from build123d import *

# Parameters (mm, degrees)
CROQUIS1_R              = 8.001
SALIENTE_EXTRUIR1_DEPTH = 31.75
SALIENTE_EXTRUIR2_DEPTH = 12.7
CROQUIS3_W              = 47.752
CROQUIS3_H              = 44.704
CORTAR_EXTRUIR4_DEPTH   = 6.35


with BuildPart() as part:
    # Croquis1 → Saliente-Extruir1 (new body)
    with BuildSketch(Plane(origin=(0, 0, 0), x_dir=(1, 0, 0), z_dir=(0, 1, 0))):
        with BuildLine():
            Line((0, -22.352), (25.4, -22.352))
            Line((25.4, -22.352), (25.4, 22.352))
            Line((25.4, 22.352), (0, 22.352))
            ThreePointArc((0, 22.352), (-22.352, 0), (0, -22.352))
        make_face()
        Circle(CROQUIS1_R, mode=Mode.SUBTRACT)
    extrude(amount=SALIENTE_EXTRUIR1_DEPTH)

    # Croquis1<3> → Saliente-Extruir2 (add)
    with BuildSketch(Plane(origin=(0, 0, 0), x_dir=(1, 0, 0), z_dir=(0, 1, 0))):
        with BuildLine():
            Line((69.85, -22.352), (69.85, -6.35))
            Line((69.85, -6.35), (57.15, -6.35))
            ThreePointArc((57.15, -6.35), (50.8, 0), (57.15, 6.35))
            Line((57.15, 6.35), (69.85, 6.35))
            Line((69.85, 6.35), (69.85, 22.352))
            Line((69.85, 22.352), (25.4, 22.352))
            Line((25.4, 22.352), (25.4, -22.352))
            Line((25.4, -22.352), (69.85, -22.352))
        make_face()
    extrude(amount=SALIENTE_EXTRUIR2_DEPTH)

    # Croquis3 → Cortar-Extruir4 (cut)
    with BuildSketch(Plane(origin=(0, 31.75, 0), x_dir=(1, 0, 0), z_dir=(0, 1, 0))):
        with Locations((1.524, 0)):
            Rectangle(CROQUIS3_W, CROQUIS3_H)
    extrude(amount=-CORTAR_EXTRUIR4_DEPTH, mode=Mode.SUBTRACT)


solid = part.part
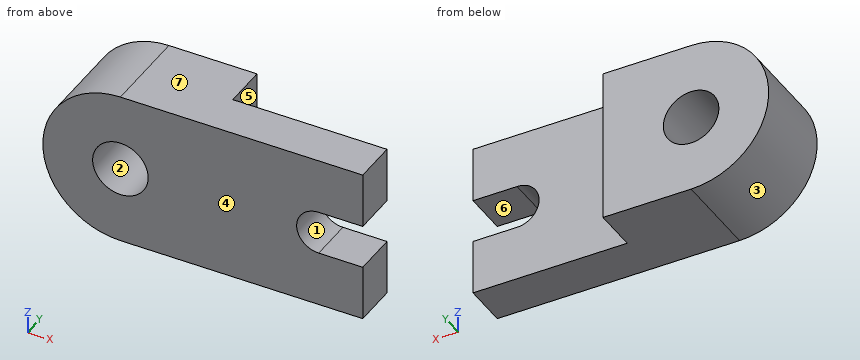
Geometry: final body of the model. Coordinates: model frame, mm. Face numbers are marked on the shaded views. A direction names the side the tool comes from. Give positions to 0.01 mm unless a question says otherwise; leave off trailing zeros. Loops run counter-clockwise (first coordinate to the right, second up) from the corner with the lowest first, then second, coordinate; pieces in that order, holes last. Notation, with made-up numbers: (19, 43.5) - (62, 43.5) arc R10 cw to (62, 56.5) - close; hole circle Ø4 at (26.25, 23.25). An arc over 180 degrees is marked (long way). Answer as CSV lines item,"result". Start each with the question number.
1. Section B-B, the plane y = 7.5. Return loops of the section in (x, z), plus the area to 3 significant figures.
2. Ray query, L1, parallel to X at y = 18.75, z = 0; L2, parallel to X at y = 7.25, z = 0; L3, parallel to Z at x = 63.5, y = 8.25. Return the intervals inside material, ascending.
3. Reachability of the marked faces 5, 6 and 7 from +Z, -Z, +X, -X, +Y, -Y: full face, straight path, thin tool, end or side. Return the list, or none.
4. Section D-D, the plane z = -9. Return loops of the section in (x, y).
5. Draft query along Z for the marked faces 1, 2, 3 and 4. Return one class per face: released by +Z, released by -Z, zero draft, split by the parting line, or undercut.
6. Section A-A, the plane z = 0. Return loops of the section in (x, y).
7. Pin query (flat end, axial travel): P1, Ø10, axis at y = 22, z = 15.5, coming from the -X side; P2, Ø6, axis at x = 48.5, z = -12, coming from the +Y side; P3, Ø4, axis at y = 20.5, z = -6.5, coming from the +X side. Return the tip coordinate at first contact, or that it passes through.
8. Section C-C, the plane x = 53.5. Return loops of the section in (y, z), plus the area to 3 significant figures.
Answers:
1,outline,"(0, -22.35) - (69.85, -22.35) - (69.85, -6.35) - (57.15, -6.35) arc R6.35 cw to (57.15, 6.35) - (69.85, 6.35) - (69.85, 22.35) - (0, 22.35) arc R22.35 ccw to start; hole circle Ø16 at (0, 0)"
1,area,"3,480 mm2"
2,L1,"x = -22.35 to -8, 8 to 25.4"
2,L2,"x = -22.35 to -8, 8 to 50.8"
2,L3,"z = -22.35 to -6.35, 6.35 to 22.35"
3,face 5,"+Z, -Z, +X, +Y"
3,face 6,"+X, +Y, -Y"
3,face 7,"+Z, +X, -X, +Y, -Y"
4,outline,"(-20.46, 0) - (69.85, 0) - (69.85, 12.7) - (25.4, 12.7) - (25.4, 25.4) - (-20.46, 25.4) - close"
5,face 1,"undercut"
5,face 2,"undercut"
5,face 3,"split by the parting line"
5,face 4,"zero draft"
6,outline,"(-22.35, 0) - (-8, 0) - (-8, 25.4) - (-22.35, 25.4) - close; (8, 0) - (50.8, 0) - (50.8, 12.7) - (25.4, 12.7) - (25.4, 25.4) - (8, 25.4) - close"
7,P1,"stops at x = -19.73"
7,P2,"stops at y = 12.7"
7,P3,"stops at x = 25.4"
8,outline,"(0, -22.35) - (12.7, -22.35) - (12.7, -5.2) - (0, -5.2) - close; (0, 5.2) - (12.7, 5.2) - (12.7, 22.35) - (0, 22.35) - close"
8,area,"436 mm2"
